Geometry check sheet. Reference: the model listing, model coordinates, mm. A direction names the side the tool comes from. Give positions to 0.01 mm unless a question says otherwise; leave off trailing zeros. Order: outer loops, then holes, each group sorted by start corner. A loop starts at its lowest first (then second) coordinate and runs counter-clockwise, first axis right, second up. Notation, with made-up numbers: M 87,-25 L 125,-25 A17 cw 125,-6 Z; hole C 19.5,-7.5 d1. An arc over 180 degrees is marked long. Answer as CSV lines item,"result". Start each with the question number.
Q1. Thickness scan on line 1 (Z direction, x = 3.55, y = 4.1); line 2 (Y direction, x = 3.25, z = 8); line 3 (Y direction, x = 5.05, z = 8). Record the ranges inside material, lowest first.
Q2. Set-up check for faces 1 (the flat face through (5, 10, 8)), 2 (the cylindrical face through (2.25, -3.15, 8.11)), 3 (the flat face through (3, 4, 16)), 4 (the flat face through (1.232, 5.53, 10.523)), 5 (the flat face through (5, -2, 8)): record each of +Z, -Z, +X, -X, +Y, -Y from which the full face is reachable in a straight line by a thin tool's end or side.
Q3. Mould release check, pull along Z, two halves, no side actions. Record for faces 6 (the flat face through (1.23, 2.63, 10.5)), 7 (the flat face through (5.5, 7.85, 8.1)), 8 (the flat face through (3, 4, 0)): +Z half, -Z half, draft (parallel to the pull), parting line (faces both ways), or undercut.
Q4. Section check A-A, the plane z = 8. Record the boundary of the cut face in (x, y), then the cut area to 3 significant figures.
Q5. Go/stop test with flat-tipped pins: pin 1 (1.2 mm diameter, centred on x = 1, z = 8.5, fed in from +Y); pin 2 (1.9 mm diameter, centred on y = 9, z = 8, fed in from +X); pin 3 (1.5 mm diameter, centred on y = 8, z = 7, fed in from +X); pin 4 (0.5 mm diameter, centred on x = 5.5, z = 10.5, fed in from -Y). Record where each tip stops, or that it passes through.
Q6. Section check B-B, the plane x = 3.9. Record the boundary of the cut face in (y, z).
Q7. Section check D-D, the plane x = 5.6. Record the boundary of the cut face in (y, z), then the cut area to 3 significant figures.
Q8. Section check C-C, the plane z = 14. Record the boundary of the cut face in (x, y).
```python
from build123d import *

# Parameters (mm, degrees)
SALIENTE_EXTRUIR1_DEPTH = 16
CROQUIS2_R              = 1.55
CORTAR_EXTRUIR1_DEPTH   = 5
CORTAR_EXTRUIR2_DEPTH   = 2.5
REDONDEO1_R             = 2
CROQUIS4_W              = 16
CROQUIS4_H              = 7.5
CROQUIS4_R              = 1.55
SALIENTE_EXTRUIR3_DEPTH = 1


with BuildPart() as part:
    # Croquis1 → Saliente-Extruir1 (new body)
    with BuildSketch(Plane.XY):
        Polygon((2.1, -3.4), (5, -3.4), (5, 11.6), (2.1, 11.6), (0, 8.2), (0, 0), align=None)
    extrude(amount=SALIENTE_EXTRUIR1_DEPTH)

    # Croquis2 → Cortar-Extruir1 (cut)
    with BuildSketch(Plane.ZY):
        with Locations(Location((8, 4.1, 0), (0, 0, 270))):
            Circle(CROQUIS2_R)
    extrude(amount=-CORTAR_EXTRUIR1_DEPTH, mode=Mode.SUBTRACT)

    # Croquis3 → Cortar-Extruir2 (cut)
    with BuildSketch(Plane.ZY):
        Polygon((11.348631561, 4.1), (9.674315781, 7), (6.325684219, 7), (4.651368439, 4.1), (6.325684219, 1.2), (9.674315781, 1.2), align=None)
    extrude(amount=-CORTAR_EXTRUIR2_DEPTH, mode=Mode.SUBTRACT)

    # Redondeo1
    redondeo1_edges = [part.edges().sort_by_distance(p)[0] for p in [
        (2.1, -3.4, 8),
        (0, 0, 8),
        (0, 8.2, 8),
        (2.1, 11.6, 8),
    ]]
    fillet(redondeo1_edges, radius=REDONDEO1_R)

    # Croquis4 → Saliente-Extruir3 (add)
    with BuildSketch(Plane(origin=(5, 0, 0), x_dir=(0, 0, -1), z_dir=(1, 0, 0))):
        with Locations((-8, 4.1)):
            Rectangle(CROQUIS4_W, CROQUIS4_H)
        with Locations(Location((-8, 4.1, 0), (0, 0, 270))):
            Circle(CROQUIS4_R, mode=Mode.SUBTRACT)
    extrude(amount=SALIENTE_EXTRUIR3_DEPTH)


solid = part.part
```
Answer block:
1,line 1,"z = 0 to 6.45, 9.55 to 16"
1,line 2,"y = -3.4 to 2.55, 5.65 to 11.6"
1,line 3,"y = 0.35 to 2.55, 5.65 to 7.85"
2,face 1,"+Z, -Z, +X, +Y"
2,face 2,"+Z, -Z, -X, -Y"
2,face 3,"+Z, +X, -X, +Y, -Y"
2,face 4,"-X"
2,face 5,"+Z, -Z, +X, -Y"
3,face 6,"undercut"
3,face 7,"draft"
3,face 8,"-Z half"
4,outline,"M 0,0.57 A2 ccw 0.3,-0.48 L 1.51,-2.45 A2 ccw 3.22,-3.4 L 5,-3.4 L 5,0.35 L 6,0.35 L 6,2.55 L 2.5,2.55 L 2.5,1.2 L 0,1.2 Z; M 0,7 L 2.5,7 L 2.5,5.65 L 6,5.65 L 6,7.85 L 5,7.85 L 5,11.6 L 3.22,11.6 A2 ccw 1.51,10.65 L 0.3,8.68 A2 ccw 0,7.63 Z"
4,area,"49.6 mm2"
5,pin 1,"stops at y = 10.78"
5,pin 2,"stops at x = 5"
5,pin 3,"stops at x = 6"
5,pin 4,"stops at y = 0.35"
6,outline,"M -3.4,0 L 11.6,0 L 11.6,16 L -3.4,16 Z; hole C 4.1,8 d3.1"
7,outline,"M 0.35,0 L 7.85,0 L 7.85,16 L 0.35,16 Z; hole C 4.1,8 d3.1"
7,area,"112 mm2"
8,outline,"M 0,0.57 A2 ccw 0.3,-0.48 L 1.51,-2.45 A2 ccw 3.22,-3.4 L 5,-3.4 L 5,0.35 L 6,0.35 L 6,7.85 L 5,7.85 L 5,11.6 L 3.22,11.6 A2 ccw 1.51,10.65 L 0.3,8.68 A2 ccw 0,7.63 Z"
